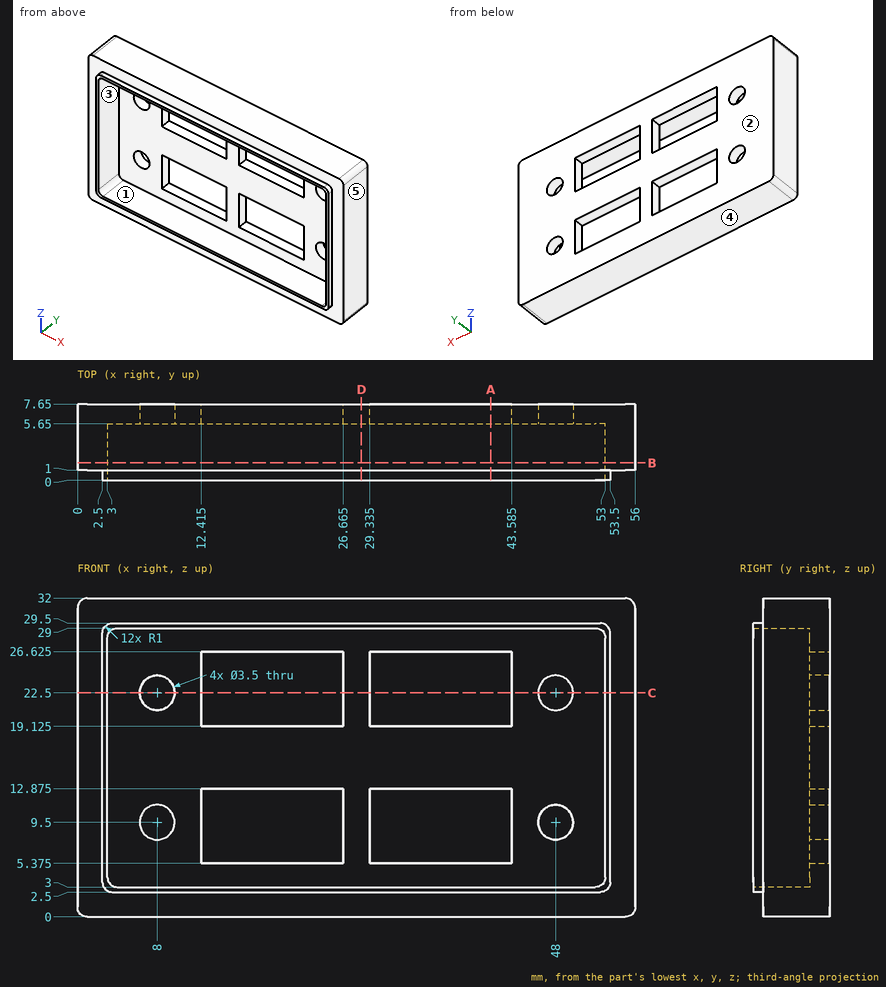
For this review, use the dimensioned drawing (mm, ordinates from the lowest corner) and the shaded views. A direction names the side the tool comes from. Coordinates: 2 decimals unless noted, no trailing zeros. Write each loop counter-clockwise with the first axis right and the second up, starting at its lowest first coordinate (ties: lowest second). Pieces come first, ordered by that corner, then holes. Notation, with made-up numbers: (75.25, 43.5) - (102.25, 43.5) arc R22 ccw to (102.25, 60.5) - close; hole circle Ø8 at (-40, 23.5). An arc over 180 degrees is marked (long way). Answer as a JSON object with one key per item and string values. Group by question number.
1. Clearance check with a flat-ended pin moving along its axis: pin 1 Ø5 at (x, z) = (42.5, 6) entering from -Y. State where the tip first meets the part, or that it passes through.
2. To check wall thickness, follow probe 1 along Z at (x, y) = (41.5, 7.25) (3 decimals); probe 2 along Z at (x, y) = (48, 6.9); probe 3 along X at (y, z) = (7.2, 9.5) (3 decimals). State the ranges of each line that lie inside material, in increasing order.
3. Mouldability with a two-part tool opening along Z and no side actions: class the marked faces 3, 4 and 5 as pulls with the +Z half, pulls with the -Z half, needs draft (parallel to the pull), parting line crosses it, or undercut.
4. Add section D-D (x = 28.5). Give the boundary of the cut face in (y, z), plus the area to 3 significant figures.
5. Add section B-B (y = 1.75). Give the boundary of the cut face in (x, z), plus the area to 3 significant figures.
6. Add section C-C (z = 22.5). Give the boundary of the cut face in (x, y) (3 decimals), plus the area to 3 significant figures.
7. Add section A-A (x = 41.5). Give the boundary of the cut face in (y, z) (3 decimals).
8. Machinability: for the marked faces 1 and 2, which of the approach directions +Z, -Z, +X, -X, +Y, -Y give a long, thin tool a straight path to every point of the face, cutting with its end or side? Answer none if there is none.
Findings:
{
 "1": {"pin 1": "y = 5.65"},
 "2": {"probe 1": "0 to 5.375, 12.875 to 19.125, 26.625 to 32", "probe 2": "0 to 7.75, 11.25 to 20.75, 24.25 to 32", "probe 3": "0 to 6.25, 9.75 to 12.415, 26.665 to 29.335, 43.585 to 46.25, 49.75 to 56"},
 "3": {"face 3": "undercut", "face 4": "pulls with the -Z half", "face 5": "needs draft"},
 "4": {"outline": "(0, 2.5) - (1, 2.5) - (1, 0) - (7.65, 0) - (7.65, 32) - (1, 32) - (1, 29.5) - (0, 29.5) - (0, 29) - (5.65, 29) - (5.65, 3) - (0, 3) - close", "area": "92.9 mm²"},
 "5": {"outline": "(0, 1) arc R1 ccw to (1, 0) - (55, 0) arc R1 ccw to (56, 1) - (56, 31) arc R1 ccw to (55, 32) - (1, 32) arc R1 ccw to (0, 31) - close; hole (3, 4) arc R1 ccw to (4, 3) - (52, 3) arc R1 ccw to (53, 4) - (53, 28) arc R1 ccw to (52, 29) - (4, 29) arc R1 ccw to (3, 28) - close", "area": "492 mm²"},
 "6": {"outline": "(0, 1) - (2.5, 1) - (2.5, 0) - (3, 0) - (3, 5.65) - (6.25, 5.65) - (6.25, 7.65) - (0, 7.65) - close; (9.75, 5.65) - (12.415, 5.65) - (12.415, 7.65) - (9.75, 7.65) - close; (26.665, 5.65) - (29.335, 5.65) - (29.335, 7.65) - (26.665, 7.65) - close; (43.585, 5.65) - (46.25, 5.65) - (46.25, 7.65) - (43.585, 7.65) - close; (49.75, 5.65) - (53, 5.65) - (53, 0) - (53.5, 0) - (53.5, 1) - (56, 1) - (56, 7.65) - (49.75, 7.65) - close", "area": "69.9 mm²"},
 "7": {"outline": "(0, 2.5) - (1, 2.5) - (1, 0) - (7.65, 0) - (7.65, 5.375) - (5.65, 5.375) - (5.65, 3) - (0, 3) - close; (0, 29) - (5.65, 29) - (5.65, 26.625) - (7.65, 26.625) - (7.65, 32) - (1, 32) - (1, 29.5) - (0, 29.5) - close; (5.65, 12.875) - (7.65, 12.875) - (7.65, 19.125) - (5.65, 19.125) - close"},
 "8": {"face 1": "-Y", "face 2": "+Z, -Z, +X, -X, +Y"}
}
